Read the model definition and answer for the solid it produces. Units are mm, in the model's axes. Face numbers are marked on the shaded views. A direction names the side the tool comes from. Round coordinates to 2 decimals unless told otherwise and drop trailing zeros. Loops run counter-clockwise (first coordinate to the right, second up) from the corner with the lowest first, then second, coordinate; pieces in that order, holes last. Notation, with made-up numbers: (-13.5, -5.5) -> (-8.5, -5.5) arc R16 cw to (-8.5, 21.5) -> close; hole circle Ø6 at (24.5, -22.75). An arc over 180 degrees is marked (long way). Put each result on its own line as item: value.
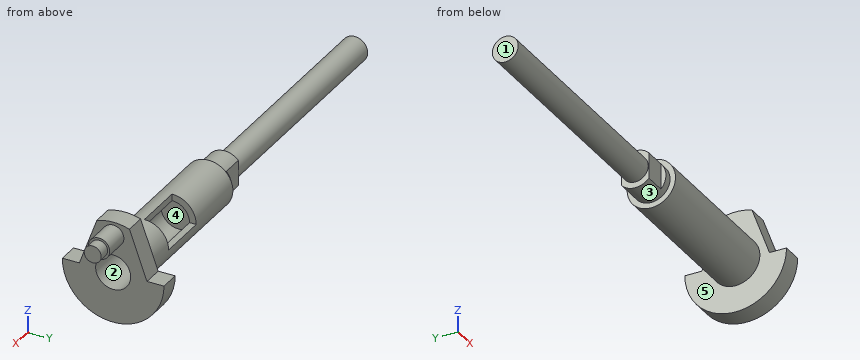
Autodesk Inventor part; units mm, degrees
ref_plane "YZ Plane" through (0, 0, 0) normal (1, 0, 0) x (0, 1, 0)
ref_plane "XZ Plane" through (0, 0, 0) normal (0, 1, 0) x (-1, 0, 0)
ref_plane "XY Plane" through (0, 0, 0) normal (0, 0, 1) x (1, 0, 0)
sketch "Sketch1" plane through (0, 0, 0) normal (1, 0, 0) x (0, 1, 0)
  circle A0 centre (0, 0) radius 9.4742
  dimension "d0" = 9.4742
extrude "Extrusion1" add sketch "Sketch1" against normal blind 3.81
sketch "Sketch2" plane through (0, 0, 0) normal (1, 0, 0) x (0, 0, -1)
  circle A0 centre (0, 0) radius 9.4742
  circle A1 centre (0, 0) radius 4.5085
  dimension "d4" = 9.017
extrude "Extrusion2" add sketch "Sketch2" against normal blind 32.639 contours A1
sketch "Sketch3" plane through (0, 0, 0) normal (1, 0, 0) x (0, 0, -1)
  circle A0 centre (0, 0) radius 9.4742
  circle A1 centre (0, 0) radius 3.4925
  dimension "d9" = 6.985
extrude "Extrusion3" add sketch "Sketch3" against normal blind 38.1 contours A1
sketch "Sketch4" plane through (0, 0, 0) normal (1, 0, 0) x (0, 0, -1)
  circle A0 centre (0, 0) radius 9.4742
  circle A1 centre (0, 0) radius 2.413
  dimension "d13" = 4.826
extrude "Extrusion4" add sketch "Sketch4" against normal blind 82.55 contours A1
sketch "Sketch5" plane through (0, 0, 0) normal (0, 0, 1) x (1, 0, 0)
  line L0 (-3.81, 9.4742) -> (0, 9.4742)
  line L1 (0, 9.4742) -> (0, -9.4742)
  line L2 (0, -9.4742) -> (-3.81, -9.4742)
  line L3 (-3.81, -9.4742) -> (-3.81, -4.5085)
  line L4 (-3.81, -4.5085) -> (-32.639, -4.5085)
  line L5 (-32.639, -4.5085) -> (-32.639, -3.4925)
  line L6 (-32.639, -3.4925) -> (-38.1, -3.4925)
  line L7 (-38.1, -3.4925) -> (-38.1, -2.413)
  line L8 (-38.1, -2.413) -> (-82.55, -2.413)
  line L9 (-82.55, -2.413) -> (-82.55, 2.413)
  line L10 (-82.55, 2.413) -> (-38.1, 2.413)
  line L11 (-38.1, 2.413) -> (-38.1, 3.4925)
  line L12 (-38.1, 3.4925) -> (-32.639, 3.4925)
  line L13 (-32.639, 3.4925) -> (-32.639, 4.5085)
  line L14 (-32.639, 4.5085) -> (-3.81, 4.5085)
  line L15 (-3.81, 4.5085) -> (-3.81, 9.4742)
  line L16 (-38.1, 3.4925) -> (-34.036, 3.4925)
  line L17 (-34.036, 3.4925) -> (-34.036, 2.54)
  line L18 (-34.036, 2.54) -> (-38.1, 2.54)
  line L19 (-38.1, 2.54) -> (-38.1, 3.4925)
  line L20 (-38.1, -3.4925) -> (-34.036, -3.4925)
  line L21 (-34.036, -3.4925) -> (-34.036, -2.54)
  line L22 (-34.036, -2.54) -> (-38.1, -2.54)
  line L23 (-38.1, -2.54) -> (-38.1, -3.4925)
  point P0 (0, 0)
  dimension "d17" = 34.036
  dimension "d18" = 5.08
extrude "Extrusion5" cut sketch "Sketch5" along normal through all both and the other way through all contours L17 L18 L11 L12 | L6 L7 L22 L21
thread "Thread1"
sketch "Sketch6" plane through (0, 0, 0) normal (1, 0, 0) x (0, 0, -1)
  circle A0 centre (0, 0) radius 9.4742
hole "Hole1" at (0, 0, 0) direction (-1, 0, 0) diameter 6.5278 depth 22.352
sketch "Sketch7" plane through (0, 0, 0) normal (0, 0, 1) x (1, 0, 0)
  line L0 (-3.81, 9.4742) -> (0, 9.4742)
  line L1 (0, 9.4742) -> (0, 3.2639)
  line L2 (0, 3.2639) -> (-22.352, 3.2639)
  line L3 (-22.352, 3.2639) -> (-22.352, -3.2639)
  line L4 (-22.352, -3.2639) -> (0, -3.2639)
  line L5 (0, -3.2639) -> (0, -9.4742)
  line L6 (0, -9.4742) -> (-3.81, -9.4742)
  line L7 (-3.81, -9.4742) -> (-3.81, -4.5085)
  line L8 (-3.81, -4.5085) -> (-32.639, -4.5085)
  line L9 (-32.639, -4.5085) -> (-32.639, -3.4925)
  line L10 (-32.639, -3.4925) -> (-34.036, -3.4925)
  line L11 (-34.036, -3.4925) -> (-34.036, -2.54)
  line L12 (-34.036, -2.54) -> (-38.1, -2.54)
  line L13 (-38.1, -2.54) -> (-38.1, -2.413)
  line L14 (-38.1, -2.413) -> (-82.55, -2.413)
  line L15 (-82.55, -2.413) -> (-82.55, 2.413)
  line L16 (-82.55, 2.413) -> (-38.1, 2.413)
  line L17 (-38.1, 2.413) -> (-38.1, 2.54)
  line L18 (-38.1, 2.54) -> (-34.036, 2.54)
  line L19 (-34.036, 2.54) -> (-34.036, 3.4925)
  line L20 (-34.036, 3.4925) -> (-32.639, 3.4925)
  line L21 (-32.639, 3.4925) -> (-32.639, 4.5085)
  line L22 (-32.639, 4.5085) -> (-3.81, 4.5085)
  line L23 (-3.81, 4.5085) -> (-3.81, 9.4742)
  line L24 (-65.532, 0) -> (10.922, 0)
  line L25 (-10.668, 0) -> (-20.1168, 0)
  line L26 (-20.1168, 0) -> (-20.1168, 4.5085)
  line L27 (-20.1168, 4.5085) -> (-10.668, 4.5085)
  line L28 (-10.668, 4.5085) -> (-10.668, 0)
  point P0 (0, 0)
  dimension "d30" = 10.668
  dimension "d31" = 20.1168
extrude "Extrusion6" cut sketch "Sketch7" along normal through all contours L28 L2 L26 L22 | L28 L24 L26 L2
sketch "Sketch8" plane through (0, 0, 0) normal (1, 0, 0) x (0, 0, -1)
  circle A0 centre (0, 0) radius 3.2639
  circle A1 centre (0, 0) radius 9.4742
  line L0 (0, -9.4742) -> (0, -6.2992)
  line L1 (0, -6.2992) -> (-8.9758, -3.0323)
  line L2 (0, 0) -> (-9.4742, 0)
  line L3 (0, 9.4742) -> (0, 6.2992)
  line L4 (0, 6.2992) -> (-8.9758, 3.0323)
  dimension "d34" = 3.175
  dimension "d36" = 110
extrude "Extrusion7" cut sketch "Sketch8" against normal through all contours A1 L3 L4 | L1 L0 A1
sketch "Sketch9" plane through (0, 0, 0) normal (1, 0, 0) x (0, 0, -1)
  arc A0 (0, -9.4742) -> (0, 9.4742) centre (0, 0) ccw
  circle A1 centre (-6.9342, 0) radius 1.9939
  dimension "d43" = 6.9342
  dimension "d47" = 3.9878
extrude "Extrusion8" add sketch "Sketch9" along normal blind 4.826
sketch "Sketch10" plane through (4.826, 0, 6.9342) normal (1, 0, 0) x (0, 0, -1)
  circle A0 centre (0, 0) radius 1.9939
  circle A1 centre (0, 0) radius 1.5875
  point P0 (6.9342, 0)
  dimension "d49" = 3.175
extrude "Extrusion9" add sketch "Sketch10" along normal blind 2.159 contours A1
properties part number "Crankshaft" material "Steel"
Item 1: The part is cut by section D-D (x = -17). Determine the outline of the cut face in (y, z), then the cut area to 3 significant figures.
Derived:
outline: (0, 3.26) -> (0, 4.51) arc R4.51 ccw (long way) to (4.51, 0) -> (3.26, 0) arc R3.26 cw (long way) to start
area: 22.8 mm^2
Item 2: The part is cut by section A-A (x = 2.5). Determine the outline of the cut face in (y, z).
Derived:
outline: circle Ø3.99 at (0, 6.93)
Item 3: Which of the six approach directions +Z, -Z, +X, -X, +Y, -Y give full straight-line access (tool end or side, diameter ignored) to the marked faces 4 and 5?
Derived:
face 4: +X
face 5: -X
Item 4: Find the intervals of material crossed by line 1 along X through (y, z) = (3.25, 1); line 2 along Z through (x, y) = (-9.25, 0); line 3 along X through (y, z) = (-1, 0.75), in increasing order.
Derived:
line 1: x = -34.04 to -20.12, -10.67 to 0
line 2: z = -4.51 to -3.26, 3.26 to 4.51
line 3: x = -82.55 to -22.35
Item 5: The part is cut by section C-C (y = -8). Determine the outline of the cut face in (x, z), then the cut area to 3 significant figures.
Derived:
outline: (-3.81, -5.08) -> (0, -5.08) -> (0, 0) -> (-3.81, 0) -> close
area: 19.3 mm^2
Item 6: Flat-ended cylindrical pins translate along their axes: pin 1 Ø1.5 at (x, z) = (-54, 1) entering from -Y; pin 2 Ø3 at (x, z) = (-72.5, -0.5) entering from +Y; pin 3 Ø0.6 at (x, y) = (-14.5, 4) entering from +Z; pin 4 Ø3 at (x, y) = (-44, -5) entering from +Z. Find the tip coordinate at first contact, or state that the pin passes through.
Derived:
pin 1: stops at y = -2.4
pin 2: stops at y = 2.41
pin 3: stops at z = 0
pin 4: passes through
Item 7: The part is cut by section B-B (z = 6.25). Determine the outline of the cut face in (x, y) (3 decimals).
Derived:
outline: (-3.81, -4.024) -> (0, -4.024) -> (0, -1.873) -> (4.826, -1.873) -> (4.826, -1.432) -> (6.985, -1.432) -> (6.985, 1.432) -> (4.826, 1.432) -> (4.826, 1.873) -> (0, 1.873) -> (0, 4.024) -> (-3.81, 4.024) -> close
Item 8: For a pull along Y with two mould halves and no side action, classify the marked faces 1, 2 and 3 as pulls with the +Y half, pulls with the -Y half, needs draft (parallel to the pull), parting line crosses it, or undercut.
Derived:
face 1: needs draft
face 2: undercut
face 3: parting line crosses it
